Geometry check sheet. Reference: the model listing, model coordinates, mm. Give positions to 0.01 mm unless a question says otherwise; leave off trailing zeros. Order: outer loops, then holes, each group sorted by start corner. A loop starts at its lowest first (then second) coordinate and runs counter-clockwise, first axis right, second up. Notation, with made-up numbers: M 56,27 L 80,27 A16 ccw 80,35 Z; hole C 20.5,-3.75 d3. An arc over 180 degrees is marked long. Answer as CSV lines item,"result". Start each with the question number.
Q1. Section check C-C, the plane x = -1.6. Record the boundary of the cut face in (y, z).
Q2. Section check A-A, the plane z = 17. Record the boundary of the cut face in (x, y), then the cut area to 3 significant figures.
Q3. Thickness scan on line 1 (Z direction, x = -2, y = 0.3); line 2 (X direction, y = 0.1, z = 14); line 3 (Y direction, x = 0, z = 14.5). Record the ranges inside material, lowest first.
Q4. Section check B-B, the plane y = 0. Record the boundary of the cut face in (x, z).
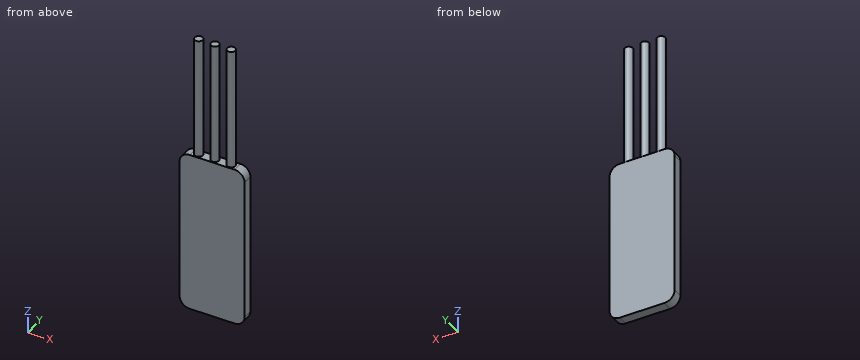
```python
from build123d import *

# Parameters (mm, degrees)
SKETCH1_W         = 6.4
SKETCH1_H         = 16
BASE_DEPTH        = 0.5
BF_R              = 1
SKETCH2_R         = 0.4
WIRE_2_DEPTH      = 12
WIRE_LP_COUNT     = 2
WIRE_LP_PITCH     = 1.6
WIRE_LP_COL_COUNT = 2
WIRE_LP_COL_PITCH = 1.6


with BuildPart() as part:
    # Sketch1 → BASE (new, symmetric)
    with BuildSketch(Plane(origin=(0, 0, 0), x_dir=(1, 0, 0), z_dir=(0, 1, 0))):
        Rectangle(SKETCH1_W, SKETCH1_H)
    extrude(amount=BASE_DEPTH, both=True)

    # BF
    bf_edges = [part.edges().sort_by_distance(p)[0] for p in [
        (3.2, 0, 8),
        (-3.2, 0, 8),
        (-3.2, 0, -8),
        (3.2, 0, -8),
    ]]
    fillet(bf_edges, radius=BF_R)

    # Sketch2 → WIRE 2 (add)
    with BuildSketch(Plane.XY.offset(8)):
        with Locations(Location((0, 0, 0), (0, 0, 180))):
            Circle(SKETCH2_R)
    wire_2 = extrude(amount=WIRE_2_DEPTH)

    # WIRE LP: WIRE 2 ×2
    with Locations(*[(-i * WIRE_LP_PITCH, 0, 0) for i in range(1, WIRE_LP_COUNT)]):
        add(wire_2)

    # WIRE LP col: WIRE 2 ×2
    with Locations(*[(i * WIRE_LP_COL_PITCH, 0, 0) for i in range(1, WIRE_LP_COL_COUNT)]):
        add(wire_2)


solid = part.part
```
Answer block:
1,outline,"M -0.5,-8 L 0.5,-8 L 0.5,8 L 0.4,8 L 0.4,20 L -0.4,20 L -0.4,8 L -0.5,8 Z"
2,outline,"C -1.6,0 d0.8; C 0,0 d0.8; C 1.6,0 d0.8"
2,area,"1.51 mm2"
3,line 1,"z = -8 to 8"
3,line 2,"x = -1.99 to -1.21, -0.39 to 0.39, 1.21 to 1.99"
3,line 3,"y = -0.4 to 0.4"
4,outline,"M -3.2,-7 A1 ccw -2.2,-8 L 2.2,-8 A1 ccw 3.2,-7 L 3.2,7 A1 ccw 2.2,8 L 2,8 L 2,20 L 1.2,20 L 1.2,8 L 0.4,8 L 0.4,20 L -0.4,20 L -0.4,8 L -1.2,8 L -1.2,20 L -2,20 L -2,8 L -2.2,8 A1 ccw -3.2,7 Z"
